Source: three-view drawing plus pictorial views. Frame: mm from the lowest corner of the part. Coordinates: 2 decimals unless noted, no trailing zeros. Write each loop counter-clockwise with the first axis right and the second up, starting at its lowest first coordinate (ties: lowest second). Pieces come first, ordered by that corner, then holes. Notation, with made-up numbers: (-17, -3.75) -> (-7, -3.75) arc R16 ccw to (-7, 13.25) -> close; hole circle Ø2 at (89.5, 45). An arc over 180 degrees is marked (long way). Write item = value, one per line.
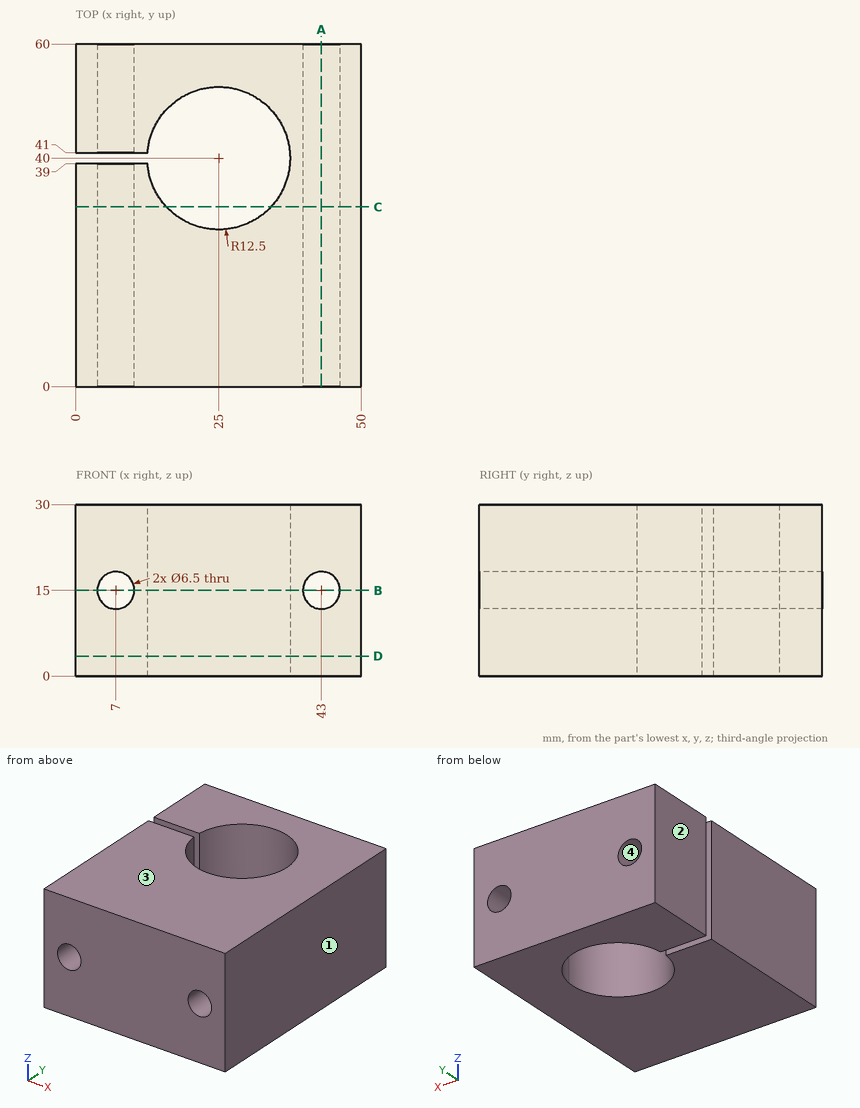
1) First-contact query: pin 1 Ø10 at (x, z) = (24.5, 20.5) entering from -Y. Flat tip, straight axial feed; report the tip coordinate or a pass-through.
Answer block:
pin_1 = 0
2) Cut plane B-B, the plane z = 15. Output: boundary loops of the cut face in (x, y).
Answer block:
outline = (0, 0) -> (3.75, 0) -> (3.75, 39) -> (0, 39) -> close; (0, 41) -> (3.75, 41) -> (3.75, 60) -> (0, 60) -> close; (10.25, 0) -> (39.75, 0) -> (39.75, 60) -> (10.25, 60) -> (10.25, 41) -> (12.54, 41) arc R12.5 cw (long way) to (12.54, 39) -> (10.25, 39) -> close; (46.25, 0) -> (50, 0) -> (50, 60) -> (46.25, 60) -> close
3) Cut plane A-A, the plane x = 43. Output: boundary loops of the cut face in (y, z).
Answer block:
outline = (0, 0) -> (60, 0) -> (60, 11.75) -> (0, 11.75) -> close; (0, 18.25) -> (60, 18.25) -> (60, 30) -> (0, 30) -> close
4) Material intervals for probe 1 along Z at (x, y) = (7, 46); probe 2 along X at (y, z) = (26, 16.75); probe 3 along X at (y, z) = (32, 23.75), sorted ascending. Write a range as [from, to].
Answer block:
probe_1 = [0, 11.75], [18.25, 30]
probe_2 = [0, 4.26], [9.74, 40.26], [45.74, 50]
probe_3 = [0, 15.4], [34.6, 50]
5) Pull-direction query (X, two-part tool) for the marked faces 1, 2, 3 and 4; classes: +X half, -X half, draft (parallel to the pull), parting line (faces both ways), or undercut.
Answer block:
face_1 = +X half
face_2 = -X half
face_3 = draft
face_4 = undercut
6) Cut plane C-C, the plane y = 31.5. Output: boundary loops of the cut face in (x, z).
Answer block:
outline = (0, 0) -> (15.83, 0) -> (15.83, 30) -> (0, 30) -> close; (34.17, 0) -> (50, 0) -> (50, 30) -> (34.17, 30) -> close; hole circle Ø6.5 at (7, 15); hole circle Ø6.5 at (43, 15)
7) Cut plane D-D, the plane z = 3.5. Output: boundary loops of the cut face in (x, y).
Answer block:
outline = (0, 0) -> (50, 0) -> (50, 60) -> (0, 60) -> (0, 41) -> (12.54, 41) arc R12.5 cw (long way) to (12.54, 39) -> (0, 39) -> close
